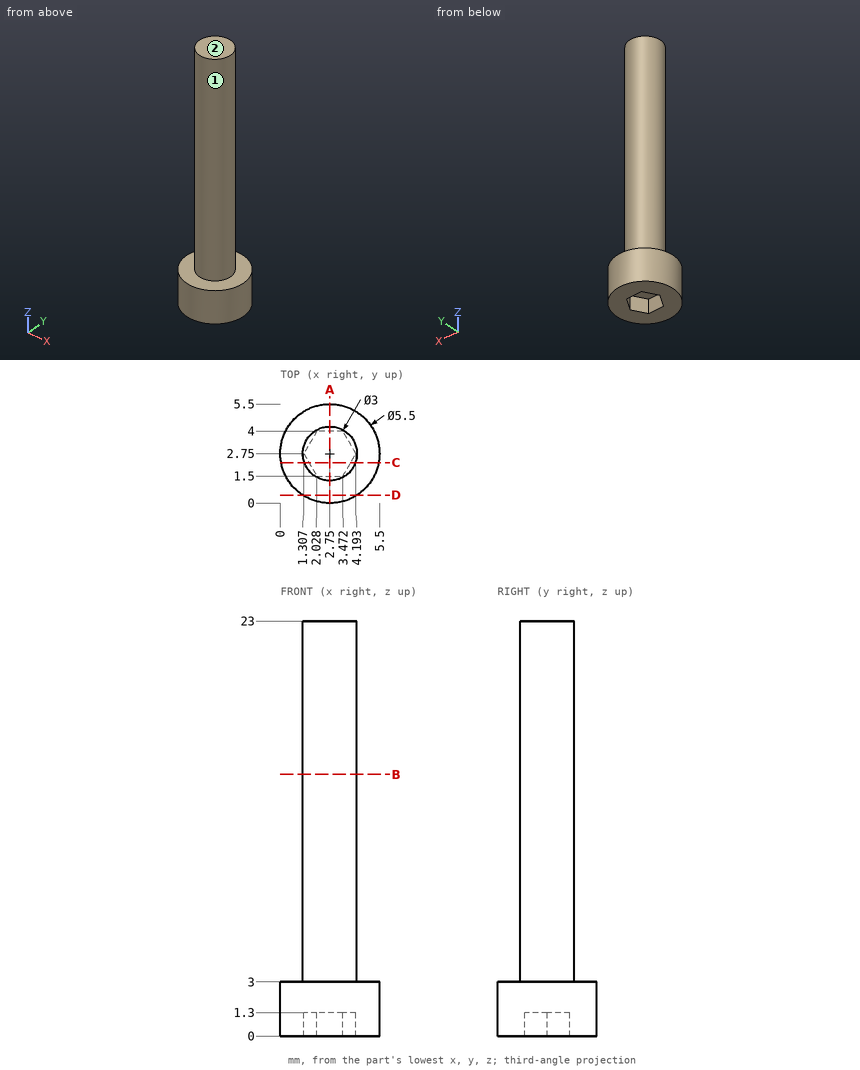
For this review, use the dimensioned drawing (mm, ordinates from the lowest corner) and the shaded views. A direction names the side the tool comes from. Round coordinates to 2 decimals unless told otherwise and drop trailing zeros. Order: outer loops, then holes, each group sorted by start corner. A loop starts at its lowest first (then second) coordinate and runs counter-clockwise, first axis right, second up. Notation, with made-up numbers: M -26.5,70.5 L 19.5,70.5 A17 cw 19.5,91.5 Z; hole C 30,3 d4. An arc over 180 degrees is marked long. Write each question's results on one line, items separated by ' | '. Start each with the question number.
1. Tool access review of the marked faces 1 and 2: name each direction out of +Z, -Z, +X, -X, +Y, -Y from which nothing blocks a thin tool from reaching the whole face with its end or side.
2. Add section A-A (x = 2.75). State the section outline as (y, z) points.
3. Add section D-D (y = 0.45). State the section outline as (x, z) points.
4. Clearance check with flat-ended pins moving along their axes: pin 1 Ø1 at (y, z) = (1, 12) entering from +X; pin 2 Ø1.4 at (x, z) = (2.5, 0.5) entering from -Y; pin 3 Ø1 at (x, z) = (3, 5.5) entering from +Y; pin 4 Ø0.8 at (x, y) = (2.5, 3) entering from -Z. State where each tip first meets the part, or that it passes through.
5. To check wall thickness, follow L1, parallel to Z at x = 4, y = 4.5; L2, parallel to Y at x = 2.75, z = 8.75; L3, parallel to X at y = 1.15, z = 1.75 (1 decimal). State the ranges of each line that lie inside material, in increasing order. Write a range as [from, to].
6. Add section B-B (z = 14.5). State the section outline as (x, y) points.
7. Add section C-C (y = 2.25). State the section outline as (x, z) points (1 decimal).
Output values:
1) face 1: +Z | face 2: +Z, +X, -X, +Y, -Y
2) outline: M 0,0 L 1.5,0 L 1.5,1.3 L 4,1.3 L 4,0 L 5.5,0 L 5.5,3 L 4.25,3 L 4.25,23 L 1.25,23 L 1.25,3 L 0,3 Z
3) outline: M 1.24,0 L 4.26,0 L 4.26,3 L 1.24,3 Z
4) pin 1: x = 3.58 | pin 2: y = 0 | pin 3: y = 4.25 | pin 4: z = 1.3
5) L1: [0, 3] | L2: [1.25, 4.25] | L3: [0.5, 5]
6) outline: C 2.75,2.75 d3
7) outline: M 0,0 L 1.6,0 L 1.6,1.3 L 3.9,1.3 L 3.9,0 L 5.5,0 L 5.5,3 L 4.2,3 L 4.2,23 L 1.3,23 L 1.3,3 L 0,3 Z
